Verification items for the finished model (mm, model axes). Face numbers are marked on the shaded views. A direction names the side the tool comes from. Round coordinates to 2 decimals unless told otherwise and drop trailing zeros. Order: outer loops, then holes, each group sorted by start corner. A loop starts at its lowest first (then second) coordinate and runs counter-clockwise, first axis right, second up. Notation, with made-up numbers: (66, 49) -> (94, 49) arc R8 ccw to (94, 56) -> close; hole circle Ø5 at (-38.75, -30). An arc over 180 degrees is marked (long way). Return JSON: item names as keys, results as strings. Group by question number.
1) Section check A-A on y = 1.5. Enter the section's corners in (x, z).
2) Depth check by flat-ended pin: pin 1 (1 mm diameter, centred on x = 22.5, y = 12, fed in from +Z); pin 2 (1.8 mm diameter, centred on y = 12, z = -18.5, fed in from -X); pin 3 (1 mm diameter, centred on x = 17.5, y = 14.5, fed in from +Z). Enter the tip coordinate at first touch or a pass-through.
3) Section check D-D on x = 8.75. Enter the section's corners in (y, z).
4) Section check C-C on y = 11.25. Enter the section's corners in (x, z).
5) Tool access check on the marked faces 1, 2 and 3. Record the directions out of +Z, -Z, +X, -X, +Y, -Y that give a thin tool (end or side, any length) a straight path to the whole face; none if there is none.
6) Section check B-B on z = -24. Enter the section's corners in (x, y).
7) Scan lines: L1, parallel to X at y = 3.6, z = -42; L2, parallel to Z at x = 15, y = 2; L3, parallel to Z at x = 5, y = 1.5. Record each from-to range of solid material in increasing order.
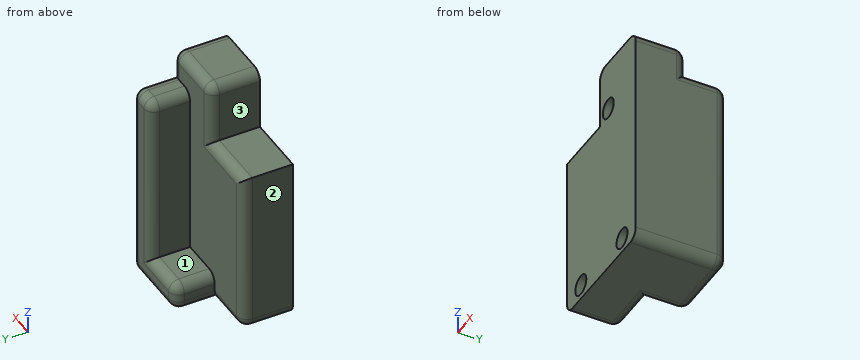
```python
from build123d import *

# Parameters (mm, degrees)
ESBO_O1_W                      = 25
ESBO_O1_H                      = 45
RESSALTO_EXTRUS_O1_DEPTH       = 10
RESSALTO_EXTRUS_O2_DEPTH       = 28
ESBO_O3_W                      = 25
ESBO_O3_H                      = 45
RESSALTO_EXTRUS_O3_DEPTH       = 6
FURO_DE_DI_METRO_4_0_4_1_D     = 4
FURO_DE_DI_METRO_4_0_4_1_DEPTH = 5
FURO_DE_DI_METRO_4_0_4_1_TIP   = 1.201721238
ESBO_O7_W                      = 10
ESBO_O7_H                      = 28
CORTE_EXTRUS_O2_DEPTH          = 5.5
ESBO_O8_W                      = 12
ESBO_O8_H                      = 12
CORTE_EXTRUS_O3_DEPTH          = 12
CORTE_EXTRUS_O4_DEPTH          = 68.720011813
FILETE2_R                      = 2


with BuildPart() as part:
    # Esboço1 → Ressalto-extrusão1 (new body)
    with BuildSketch(Plane(origin=(0, 0, 0), x_dir=(1, 0, 0), z_dir=(0, 1, 0))):
        with Locations((12.5, 22.5)):
            Rectangle(ESBO_O1_W, ESBO_O1_H)
    extrude(amount=RESSALTO_EXTRUS_O1_DEPTH)

    # Esboço2 → Ressalto-extrusão2 (add)
    with BuildSketch(Plane(origin=(0, 10, 0), x_dir=(1, 0, 0), z_dir=(0, 1, 0))):
        Polygon((0, 39.5), (19, 39.5), (19, 5.5), (0, 5.5), (0, 0), (25, 0), (25, 39.5), (25, 45), (0, 45), align=None)
    extrude(amount=RESSALTO_EXTRUS_O2_DEPTH)

    # Esboço3 → Ressalto-extrusão3 (add)
    with BuildSketch(Plane(origin=(0, 38, 0), x_dir=(1, 0, 0), z_dir=(0, 1, 0))):
        with Locations((12.5, 22.5)):
            Rectangle(ESBO_O3_W, ESBO_O3_H)
    extrude(amount=RESSALTO_EXTRUS_O3_DEPTH)

    # Furo de diâmetro Ø4.0 (4)1
    with Locations(Plane(origin=(15, 0, -10), x_dir=(0, 0, -1), z_dir=(0, -1, 0))):
        with Locations((0, 0), (32, 5), (32, -10)):
            Hole(FURO_DE_DI_METRO_4_0_4_1_D / 2, depth=FURO_DE_DI_METRO_4_0_4_1_DEPTH)
            with Locations((0, 0, -(FURO_DE_DI_METRO_4_0_4_1_DEPTH + FURO_DE_DI_METRO_4_0_4_1_TIP / 2))):  # 118° drill point
                Cone(0, FURO_DE_DI_METRO_4_0_4_1_D / 2, FURO_DE_DI_METRO_4_0_4_1_TIP, mode=Mode.SUBTRACT)

    # Esboço7 → Corte-extrusão2 (cut)
    with BuildSketch(Plane(origin=(0, 0, -45), x_dir=(-1, 0, 0), z_dir=(0, 0, -1))):
        with Locations((-5, 24)):
            Rectangle(ESBO_O7_W, ESBO_O7_H)
    extrude(amount=-CORTE_EXTRUS_O2_DEPTH, mode=Mode.SUBTRACT)

    # Esboço8 → Corte-extrusão3 (cut)
    with BuildSketch(Plane.ZY):
        with Locations((-6, 6)):
            Rectangle(ESBO_O8_W, ESBO_O8_H)
    extrude(amount=-CORTE_EXTRUS_O3_DEPTH, mode=Mode.SUBTRACT)

    # Esboço9 → Corte-extrusão4 (cut, through all)
    with BuildSketch(Plane.ZY):
        Polygon((-45, 44), (-45, 18), (-5.5, 18), (-5.5, 10), (0, 10), (0, 44), align=None)
    extrude(amount=-CORTE_EXTRUS_O4_DEPTH, mode=Mode.SUBTRACT)

    # Filete2
    filete2_edges = [part.edges().sort_by_distance(p)[0] for p in [
        (10, 14, -45),
        (10, 18, -42.25),
        (25, 9, -45),
        (25, 5, 0),
        (22, 18, -5.5),
        (19, 18, -22.5),
        (14.5, 18, -39.5),
        (25, 18, -25.25),
        (19, 14, -5.5),
        (25, 14, -5.5),
        (25, 10, -2.75),
        (18.5, 10, 0),
        (17.5, 18, -45),
        (0, 5, -45),
        (5, 10, -45),
        (10, 14, -39.5),
        (0, 10, -28.5),
        (6, 10, -12),
        (12, 5, 0),
        (12, 10, -6),
    ]]
    fillet(filete2_edges, radius=FILETE2_R)


solid = part.part
```
Check result:
{
 "1": {"outline": "(0, -43) arc R2 ccw to (2, -45) -> (23, -45) arc R2 ccw to (25, -43) -> (25, -2) arc R2 ccw to (23, 0) -> (14, 0) arc R2 ccw to (12, -2) -> (12, -12) -> (0, -12) -> close; hole circle Ø4 at (5, -42); hole circle Ø4 at (15, -10); hole circle Ø4 at (20, -42)"},
 "2": {"pin 1": "z = -5.5", "pin 2": "x = 19", "pin 3": "z = -39.5"},
 "3": {"outline": "(0, -45) -> (8, -45) arc R2 ccw to (10, -43) -> (10, -14) arc R2 ccw to (8, -12) -> (0, -12) -> close"},
 "4": {"outline": "(10, -43) arc R2 ccw to (12, -45) -> (23, -45) arc R2 ccw to (25, -43) -> (25, -7.5) arc R2 ccw to (23, -5.5) -> (21, -5.5) arc R2 ccw to (19, -7.5) -> (19, -39.5) -> (12, -39.5) arc R2 ccw to (10, -41.5) -> close"},
 "5": {"face 1": "+Z, -X, +Y", "face 2": "+Z, -Z, -X, +Y, -Y", "face 3": "+Z, -X, +Y, -Y"},
 "6": {"outline": "(0, 0) -> (25, 0) -> (25, 16) arc R2 ccw to (23, 18) -> (21, 18) arc R2 ccw to (19, 16) -> (19, 10) -> (2, 10) arc R2 ccw to (0, 8) -> close"},
 "7": {"L1": "0 to 3, 7 to 18, 22 to 25", "L2": "-45 to -12, -8 to 0", "L3": "-45 to -44, -40 to -12"}
}
